from build123d import *

# Parameters (mm, degrees)
SKETCH_4_R               = 2
SKETCH_5_R               = 0.3
CUT_EXTRUDE_1_DEPTH      = 21.95530959
PATTERN_CIRCULAR_6_COUNT = 2
PATTERN_CIRCULAR_6_ANGLE = 90
FILLET_1_R               = 0.5
CHAMFER_1_SIZE           = 0.5679439
CHAMFER_1_SIZE_2         = 0.5
FILLET_2_R               = 0.5


with BuildPart() as part:
    # Эскиз1 → Повернуть31 (revolve)
    with BuildSketch(Plane.XY, mode=Mode.PRIVATE) as revolve_31_sk:
        Polygon((0, 0), (0, 5.5), (7, 5.5), (7, 5.25), (9, 5.25), (9, 6.25), (10.5, 6.25), (10.5, 5), (19, 5), (19, 0), align=None)
    revolve(revolve_31_sk.sketch.rotate(Axis((-6.646654946, 0, 0), (1, 0, 0)), 90), axis=Axis((-6.646654946, 0, 0), (1, 0, 0)))

    # Эскиз2 → Вырез-Повернуть2 (revolve, cut)
    with BuildSketch(Plane.XY, mode=Mode.PRIVATE) as cut_revolve_2_sk:
        with BuildLine():
            Line((0, 0), (19, 0))
            Line((19, 0), (19, 4))
            Line((19, 4), (6.320642864, 2.555369732))
            Line((6.320642864, 2.555369732), (6, 2))
            Line((6, 2), (4, 2))
            ThreePointArc((4, 2), (2.401923789, 4.035898385), (0, 5))
            Line((0, 5), (0, 0))
        make_face()
    revolve(cut_revolve_2_sk.sketch.rotate(Axis((0, 0, 0), (1, 0, 0)), 90), axis=Axis((0, 0, 0), (1, 0, 0)), mode=Mode.SUBTRACT)

    # Эскиз4 → Вырез-Повернуть3 (revolve, cut)
    with BuildSketch(Plane.XY, mode=Mode.PRIVATE) as cut_revolve_3_sk:
        with Locations((4.5, 5.5)):
            Circle(SKETCH_4_R)
    revolve(cut_revolve_3_sk.sketch.rotate(Axis((0, 0, 0), (1, 0, 0)), 90), axis=Axis((0, 0, 0), (1, 0, 0)), mode=Mode.SUBTRACT)

    # Эскиз5 → Вырез-Вытянуть1 (cut, symmetric)
    with BuildSketch(Plane.XY):
        with Locations(Location((4.5, 0, 0), (0, 0, 180))):
            Circle(SKETCH_5_R)
    cut_extrude_1 = extrude(amount=CUT_EXTRUDE_1_DEPTH, both=True, mode=Mode.SUBTRACT)

    # Круговой массив6: Вырез-Вытянуть1 ×2 about axis
    pattern_circular_6_axis = Axis((-6.646654946, 0, 0), (-1, 0, 0))
    for i in range(1, PATTERN_CIRCULAR_6_COUNT):
        add(cut_extrude_1.rotate(pattern_circular_6_axis, i * PATTERN_CIRCULAR_6_ANGLE / (PATTERN_CIRCULAR_6_COUNT - 1)), mode=Mode.SUBTRACT)

    # Скругление1
    fillet_1_edges = [part.edges().sort_by_distance(p)[0] for p in [
        (19, 0, -5),
    ]]
    fillet(fillet_1_edges, radius=FILLET_1_R)

    # Фаска1
    # the kernel refuses this chamfer: 0.5679439, 0.5 mm, written as the material it takes off along each edge
    with BuildSketch(Plane(origin=(19, 0, 0), x_dir=(0, 0, 1), z_dir=(0, 1, 0))) as chamfer_1_piece_1:
        Polygon((4 + CHAMFER_1_SIZE, 0), (4 - CHAMFER_1_SIZE_2 * 0.113203213768, -CHAMFER_1_SIZE_2 * 0.993571855677), (4, 0), align=None)
    revolve(axis=Axis((19, 0, 0), (1, 0, 0)), mode=Mode.SUBTRACT)

    # Скругление2
    fillet_2_edges = [part.edges().sort_by_distance(p)[0] for p in [
        (6.320642864, 0, -2.555369732),
    ]]
    fillet(fillet_2_edges, radius=FILLET_2_R)


solid = part.part
Could you check a few things on this model? Use its own coordinates, in mm. A direction names the side the tool comes from. Coordinates: 2 decimals unless noted, no trailing zeros. Order: outer loops, then holes, each group sorted by start corner. A loop starts at its lowest first (then second) coordinate and runs counter-clockwise, first axis right, second up.
Q1. Suppose I cut it at D-D on x = 11.25. Please give me the cut outline in (y, z), and give its area (3 significant figures).
Q2. Which directions (+Z, -Z, +X, -X, +Y, -Y) give clear straight access to the entire face, cutting with the end or side of a thin tool? Please do faces 1 (the cylindrical face through (8, -1.6, 5)), 2 (the cylindrical face through (6.75, 5.37, -1.19)), 3 (the cylindrical face through (15, 0, -5)).
Q3. Please list where these lines run through material, in increasing order: L1, parallel to Y at x = 4.5, z = 2.6; L2, parallel to X at y = 4, z = 2.5; L3, parallel to Y at x = 4.5, z = -3.
Q4. Suppose I cut it at A-A on y = 0. Give the number of separate pieces and of enclosed holes in the cut face, and give its area (3 significant figures).
Q5. Suppose I cut it at B-B on x = 4.5. Please give me the cut outline in (y, z), and give its area (3 significant figures).
Q6. Thinking about a two-plate mould opening in Y: for faces 4 (the conical face through (12.454, -0.977, 3.104)), 5 (the flat face through (0, 4.9, -1.6)), 6 (the cylindrical face through (4.986, 0.766, 1.847)), 7 (the cylindrical face through (9.76, -1.88, 5.96)), which applies, released by +Y, released by -Y, zero draft, split by the parting line, or undercut?
Q7. Will these pins go through, and if not, where does the flat tip stop? pin 1 (2 mm diameter, centred on x = 15.5, y = 3, fed in from +Z); pin 2 (2 mm diameter, centred on x = 12.5, y = 0, fed in from +Z); pin 3 (1 mm diameter, centred on x = 4, y = -3.5, fed in from -Z).
Answer:
1. outline: circle Ø10 at (0, 0); hole circle Ø6.23 at (0, 0)
1. area: 48.0 mm2
2. face 1: none
2. face 2: -X
2. face 3: +X
3. L1: y = -2.34 to -0.3, 0.3 to 2.34
3. L2: x = 1.16 to 2.66, 6.34 to 18.95
3. L3: y = -1.8 to -0.3, 0.3 to 1.8
4. separate pieces: 4
4. enclosed holes: 0
4. area: 61.9 mm2
5. outline: (-3.49, -0.3) arc R3.5 ccw to (-0.3, -3.49) - (-0.3, -1.98) arc R2 cw to (-1.98, -0.3) - close; (-3.49, 0.3) - (-1.98, 0.3) arc R2 cw to (-0.3, 1.98) - (-0.3, 3.49) arc R3.5 ccw to start; (0.3, -3.49) arc R3.5 ccw to (3.49, -0.3) - (1.98, -0.3) arc R2 cw to (0.3, -1.98) - close; (0.3, 1.98) arc R2 cw to (1.98, 0.3) - (3.49, 0.3) arc R3.5 ccw to (0.3, 3.49) - close
5. area: 22.3 mm2
6. face 4: undercut
6. face 5: zero draft
6. face 6: undercut
6. face 7: split by the parting line
7. pin 1: stops at z = 4.58
7. pin 2: stops at z = 5
7. pin 3: stops at z = -1.97
